Geometry: final body of the model. Coordinates: model frame, mm. A direction names the side the tool comes from. Round coordinates to 2 decimals unless told otherwise and drop trailing zeros. Loops run counter-clockwise (first coordinate to the right, second up) from the corner with the lowest first, then second, coordinate; pieces in that order, holes last. Notation, with made-up numbers: (-27.5, 32.5) - (13.5, 32.5) arc R30 ccw to (13.5, 65.5) - close; hole circle Ø3 at (11.25, -21). An arc over 180 degrees is marked (long way). Answer in a Markdown table with one row per item. Add a question column.
from build123d import *

# Parameters (mm, degrees)
SKETCH1_W           = 160
SKETCH1_H           = 10
SKETCH1_W_2         = 9.192388155
BOSS_EXTRUDE1_DEPTH = 15
CUT_EXTRUDE1_REACH  = 205.486
SKETCH2_R           = 3.25
SKETCH2_R_2         = 1.75
FILLET1_R           = 10
SKETCH2_3_W         = 15
SKETCH2_3_H         = 5
CUT_EXTRUDE2_DEPTH  = 5
SKETCH2_4_R         = 3.25
SKETCH2_4_R_2       = 1.75
BOSS_EXTRUDE2_DEPTH = 5


with BuildPart() as part:
    # Sketch1 → Boss-Extrude1 (new body)
    with BuildSketch(Plane(origin=(0, 0, 0), x_dir=(0, 0, -1), z_dir=(1, 0, 0))):
        Polygon((113.13708499, 123.13708499), (0, 10), (14.142135624, 10), (120.208152802, 116.066017178), align=None)
        with Locations((80, 5)):
            Rectangle(SKETCH1_W, SKETCH1_H)
        with Locations((-4.596194077, 5)):
            Rectangle(SKETCH1_W_2, SKETCH1_H)
        Polygon((0, 10), (-9.192388155, 19.192388155), (-9.192388155, 10), align=None)
        Polygon((-9.192388155, 0), (-9.192388155, 10), (-9.192388155, 19.192388155), (-19.192388155, 19.192388155), (-19.192388155, 0), align=None)
    extrude(amount=BOSS_EXTRUDE1_DEPTH)

    # Sketch2 → Cut-Extrude1 (cut, up to next)
    with BuildSketch(Plane(origin=(0, 5, 5), x_dir=(1, 0, 0), z_dir=(0, 0.7071067811865562, 0.7071067811865389)), mode=Mode.PRIVATE) as cut_extrude1_sk1:
        with Locations(Location((7.5, 157.071067812, 0), (0, 0, 270))):
            Circle(SKETCH2_R)
        with Locations((7.5, 157.071067812)):
            Circle(SKETCH2_R_2, mode=Mode.SUBTRACT)
    cut_extrude1_tool1 = extrude(cut_extrude1_sk1.sketch, amount=-CUT_EXTRUDE1_REACH, mode=Mode.PRIVATE) & part.part
    # Sketch2 → Cut-Extrude1 (cut, up to next)
    with BuildSketch(Plane(origin=(0, 5, 5), x_dir=(1, 0, 0), z_dir=(0, 0.7071067811865562, 0.7071067811865389)), mode=Mode.PRIVATE) as cut_extrude1_sk2:
        with Locations((7.5, 157.071067812)):
            Circle(SKETCH2_R_2)
    cut_extrude1_tool2 = extrude(cut_extrude1_sk2.sketch, amount=-CUT_EXTRUDE1_REACH, mode=Mode.PRIVATE) & part.part
    # Sketch2 → Cut-Extrude1 (cut, up to next)
    with BuildSketch(Plane(origin=(0, 5, 5), x_dir=(1, 0, 0), z_dir=(0, 0.7071067811865562, 0.7071067811865389)), mode=Mode.PRIVATE) as cut_extrude1_sk3:
        with Locations(Location((7.5, 87.071067812, 0), (0, 0, 270))):
            Circle(SKETCH2_R)
        with Locations((7.5, 87.071067812)):
            Circle(SKETCH2_R_2, mode=Mode.SUBTRACT)
    cut_extrude1_tool3 = extrude(cut_extrude1_sk3.sketch, amount=-CUT_EXTRUDE1_REACH, mode=Mode.PRIVATE) & part.part
    # Sketch2 → Cut-Extrude1 (cut, up to next)
    with BuildSketch(Plane(origin=(0, 5, 5), x_dir=(1, 0, 0), z_dir=(0, 0.7071067811865562, 0.7071067811865389)), mode=Mode.PRIVATE) as cut_extrude1_sk4:
        with Locations((7.5, 87.071067812)):
            Circle(SKETCH2_R_2)
    cut_extrude1_tool4 = extrude(cut_extrude1_sk4.sketch, amount=-CUT_EXTRUDE1_REACH, mode=Mode.PRIVATE) & part.part
    add(cut_extrude1_tool1.solids().sort_by_distance((7.5, 118.299114, -108.299114))[0], mode=Mode.SUBTRACT)
    add(cut_extrude1_tool2.solids().sort_by_distance((7.5, 116.066017, -106.066017))[0], mode=Mode.SUBTRACT)
    add(cut_extrude1_tool3.solids().sort_by_distance((7.5, 68.80164, -58.80164))[0], mode=Mode.SUBTRACT)
    add(cut_extrude1_tool4.solids().sort_by_distance((7.5, 66.568542, -56.568542))[0], mode=Mode.SUBTRACT)

    # Fillet1
    # the kernel refuses this fillet: 10 mm, written as the material it adds along each edge
    with BuildSketch(Plane(origin=(0, 10, -14.142135624), x_dir=(0, 0.707106781186544, -0.7071067811865511), z_dir=(1, 0, 0))) as fillet1_piece_1:
        with BuildLine():
            CenterArc((FILLET1_R * 2.41421356237, -FILLET1_R), FILLET1_R, 90, 135)
            Line((FILLET1_R * 1.70710678119, -FILLET1_R * 1.70710678119), (0, 0))
            Line((0, 0), (FILLET1_R * 2.41421356237, 0))
        make_face()
    extrude(amount=15)
    # the kernel refuses this fillet: 10 mm, written as the material it takes off along each edge
    with BuildSketch(Plane(origin=(-25, 116.066017178, -120.208152802), x_dir=(0, 0.7071067811865482, 0.7071067811865468), z_dir=(1, 0, 0))) as fillet1_2_piece_1:
        with BuildLine():
            CenterArc((FILLET1_R, FILLET1_R), FILLET1_R, 180, 90)
            Line((0, FILLET1_R), (0, 0))
            Line((0, 0), (FILLET1_R, 0))
        make_face()
    extrude(amount=65, mode=Mode.SUBTRACT)
    with BuildSketch(Plane(origin=(-25, 10, -160), x_dir=(0, -1, 0), z_dir=(1, 0, 0)), Plane(origin=(-25, 19.192388155, 19.192388155), x_dir=(0, 0, -1), z_dir=(1, 0, 0))) as fillet1_2_piece_2:
        with BuildLine():
            CenterArc((FILLET1_R, -FILLET1_R), FILLET1_R, 90, 90)
            Line((0, -FILLET1_R), (0, 0))
            Line((0, 0), (FILLET1_R, 0))
        make_face()
    extrude(amount=65, mode=Mode.SUBTRACT)

    # Sketch2<3> → Cut-Extrude2 (cut)
    with BuildSketch(Plane(origin=(0, 5, 5), x_dir=(1, 0, 0), z_dir=(0, 0.7071067811865562, 0.7071067811865389))):
        with Locations((7.5, 133.571067812)):
            Rectangle(SKETCH2_3_W, SKETCH2_3_H)
        with Locations((7.5, 40.571067812)):
            Rectangle(SKETCH2_3_W, SKETCH2_3_H)
    extrude(amount=-CUT_EXTRUDE2_DEPTH, mode=Mode.SUBTRACT)

    # Sketch2<4> → Boss-Extrude2 (add)
    # profile 1 of 2: a face of its own
    with BuildSketch(Plane(origin=(0, 5, 5), x_dir=(1, 0, 0), z_dir=(0, 0.7071067811865562, 0.7071067811865389))):
        with Locations(Location((7.5, 87.071067812, 0), (0, 0, 270))):
            Circle(SKETCH2_4_R)
        with Locations(Location((7.5, 87.071067812, 0), (0, 0, 270))):
            Circle(SKETCH2_4_R_2, mode=Mode.SUBTRACT)
    # profile 2 of 2: a face of its own
    with BuildSketch(Plane(origin=(0, 5, 5), x_dir=(1, 0, 0), z_dir=(0, 0.7071067811865562, 0.7071067811865389))):
        with Locations(Location((7.5, 157.071067812, 0), (0, 0, 270))):
            Circle(SKETCH2_4_R)
        with Locations(Location((7.5, 157.071067812, 0), (0, 0, 270))):
            Circle(SKETCH2_4_R_2, mode=Mode.SUBTRACT)
    extrude(amount=-BOSS_EXTRUDE2_DEPTH)


solid = part.part
1) Reachability of faces 5 (the flat face through (7.4, 30.18, -27.25)), 6 (the cylindrical face through (7.4, 16.33, -28.98)), 7 (the flat face through (6.1, 111.54, -108.61)) from +Z, -Z, +X, -X, +Y, -Y: full face, straight path, thin tool, end or side. Return the list, or none.
2) Contact query for flat-ended pins moving along their axis: pin 1 Ø5 at (x, z) = (2, -131.5) entering from +Y; pin 2 Ø6 at (x, y) = (5.5, 22.5) entering from +Z; pin 3 Ø8 at (x, z) = (8, -86.5) entering from +Y. Output: stop coordinate, or through.
3) Pull-direction query (Y, two-part tool) for faces 1 (the flat face through (7, 21, -11)), 2 (the flat face through (0, 55, -54)), 3 (the flat face through (7, 10, -93)), 4 (the flat face through (7, 0, -69)); classes: pulls with the +Y half, pulls with the -Y half, needs draft (parallel to the pull), parting line crosses it, or undercut.
4) Section B-B, the plane z = -145. Return the cut outline in (x, y), and give its area (3 significant figures).
5) Section A-A, the plane z = -83.5. Return the cut outline in (x, y).
6) Material intervals for line 1 along Y through (x, z) = (11.25, -93.5); line 2 along Y through (x, z) = (11, -48); line 3 along Y through (x, z) = (3.75, -27.5), sorted ascending. Write a range as from..to.
7) Section C-C, the plane y = 75.5. Return the cut outline in (x, z), and give its area (3 significant figures).
Evaluation:
| question | item | result |
|---|---|---|
| 1 | face 5 | +X, -X |
| 1 | face 6 | -Z, +X, -X |
| 1 | face 7 | none |
| 2 | pin 1 | stops at y = 10 |
| 2 | pin 2 | stops at z = -9.5 |
| 2 | pin 3 | stops at y = 97.68 |
| 3 | face 1 | pulls with the +Y half |
| 3 | face 2 | needs draft |
| 3 | face 3 | undercut |
| 3 | face 4 | pulls with the -Y half |
| 4 | outline | (0, 0) - (15, 0) - (15, 10) - (0, 10) - close |
| 4 | area | 150 mm² |
| 5 | outline | (0, 0) - (15, 0) - (15, 10) - (0, 10) - close; (0, 79.36) - (15, 79.36) - (15, 93.5) - (0, 93.5) - close |
| 6 | line 1 | y = 0..10, 89.36..96.43, 98.93..103.5 |
| 6 | line 2 | y = 0..10, 43.86..58 |
| 6 | line 3 | y = 0..30.43, 33.41..37.5 |
| 7 | outline | (0, -79.64) - (15, -79.64) - (15, -65.5) - (0, -65.5) - close |
| 7 | area | 212 mm² |
